from build123d import *

# Parameters (mm, degrees)
F0_W     = 100
F0_H     = 100
F1_DEPTH = 100
F2_W     = 45.6354245543
F2_H     = 39.2044447362
F3_DEPTH = 154


# Not quite as in the source:
# - a feature names something its author has since deleted; it is built from what else it names


with BuildPart() as f1:
    # F0 (on Top) → F1 (new body)
    with BuildSketch(Plane.XY):
        with Locations((50, 50)):
            Rectangle(F0_W, F0_H)
    extrude(amount=F1_DEPTH)

    # F2 (on face) → F3 (join)
    with BuildSketch(Plane.XY.offset(100)):
        with Locations((47.8344149888, 49.6286619455)):
            Rectangle(F2_W, F2_H)
    extrude(amount=-F3_DEPTH)


solid = f1.part
For this review, take the finished solid that the model builds, in its own axes (mm). A direction names the side the tool comes from. Give positions to 0.01 mm unless a question says otherwise; leave off trailing zeros. Loops run counter-clockwise (first coordinate to the right, second up) from the corner with the lowest first, then second, coordinate; pieces in that order, holes last. Notation, with made-up numbers: (58, -37.5) -> (86, -37.5) arc R17 ccw to (86, -27.5) -> close; hole circle Ø6 at (-20.5, 82.25). An arc over 180 degrees is marked (long way). One line per question, with ' | ' between items.
1) We need section D-D (x = 87.5). Write out the cut boundary in (y, z), plus the area to 3 significant figures.
Resolved:
outline: (0, 0) -> (100, 0) -> (100, 100) -> (0, 100) -> close | area: 10,000 mm2
2) For faces 1 (the flat face through (48, 30.026, -27)), 2 (the flat face through (70.652, 49, -27)), 3 (the flat face through (25.017, 49, -27)), 4 (the flat face through (48, 69.231, -27)), list the 3-axis set-ups (+Z, -Z, +X, -X, +Y, -Y) from which the entire face can be reached by the end or side of a thin tool; tool diameter is ignored.
Resolved:
face 1: -Z, +X, -X, -Y | face 2: -Z, +X, +Y, -Y | face 3: -Z, -X, +Y, -Y | face 4: -Z, +X, -X, +Y
3) To check wall thickness, follow probe 1 along Z at (x, y) = (23, 38.5); probe 2 along Y at (x, z) = (61, -24). State the ranges of each line that lie inside material, in increasing order.
Resolved:
probe 1: z = 0 to 100 | probe 2: y = 30.03 to 69.23
4) We need section C-C (z = -24). Write out the cut boundary in (x, y), plus the area to 3 significant figures.
Resolved:
outline: (25.02, 30.03) -> (70.65, 30.03) -> (70.65, 69.23) -> (25.02, 69.23) -> close | area: 1,790 mm2
5) We need section B-B (y = 45.5). Write out the cut boundary in (x, z), plus the area to 3 significant figures.
Resolved:
outline: (0, 0) -> (25.02, 0) -> (25.02, -54) -> (70.65, -54) -> (70.65, 0) -> (100, 0) -> (100, 100) -> (0, 100) -> close | area: 12,500 mm2
6) We need section A-A (x = 35). Write out the cut boundary in (y, z), plus the area to 3 significant figures.
Resolved:
outline: (0, 0) -> (30.03, 0) -> (30.03, -54) -> (69.23, -54) -> (69.23, 0) -> (100, 0) -> (100, 100) -> (0, 100) -> close | area: 12,100 mm2
7) Insertion check: pin 1 Ø6 at (x, y) = (15.5, 80) entering from -Z; pin 2 Ø8 at (y, z) = (57.5, -20.5) entering from -X; pin 3 Ø4 at (x, z) = (68.5, -19) entering from +Y. Each pin has a flat end and moves straight along its axis. Give the tip position at first contact, or say it passes through.
Resolved:
pin 1: stops at z = 0 | pin 2: stops at x = 25.02 | pin 3: stops at y = 69.23
8) The part is to be moulded in two halves that separate along Z. For faces 5 (the flat face through (49, 51, 100)), 6 (the flat face through (48, 50, -54)), 7 (the flat face through (49, 0, 49)), say which applies: +Z half, -Z half, draft (parallel to the pull), parting line (faces both ways), or undercut.
Resolved:
face 5: +Z half | face 6: -Z half | face 7: draft
